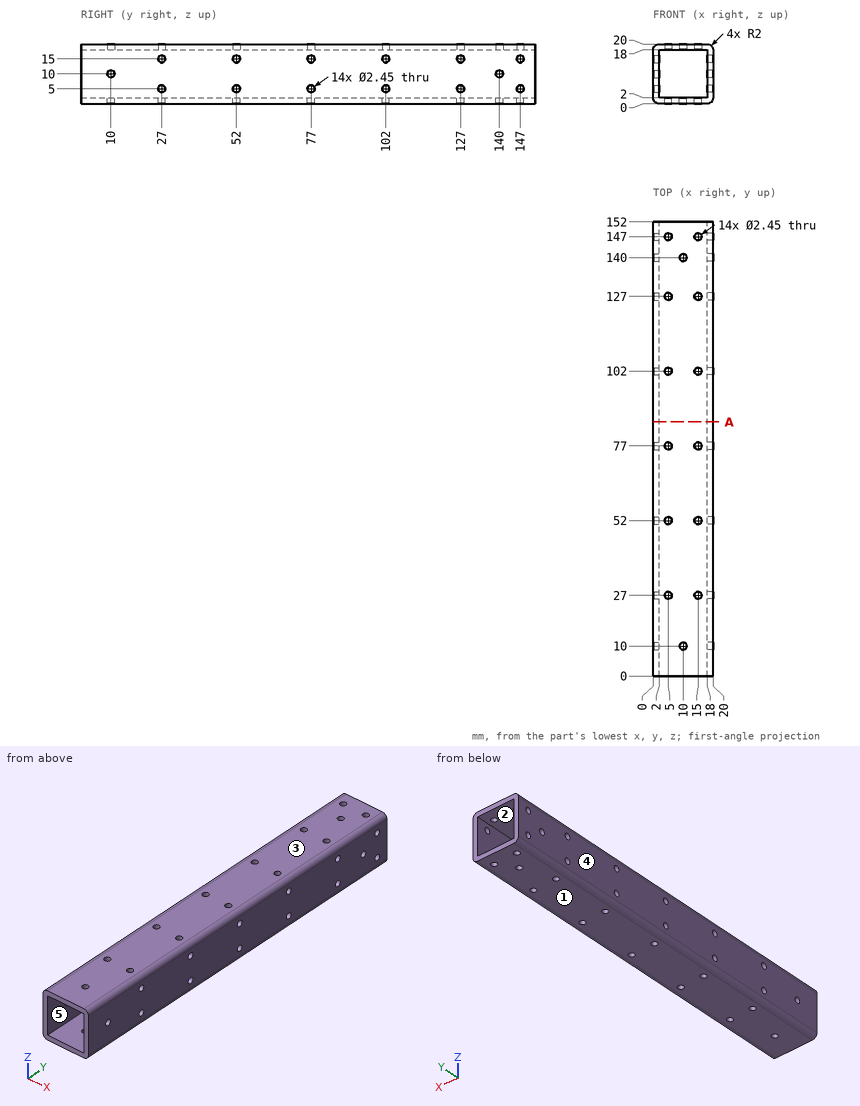
Study the drawing (mm; zero at the part's minimum x, y, z) and answer. A direction names the side the tool comes from. Coordinates: 2 decimals unless noted, no trailing zeros. Write each loop counter-clockwise with the first axis right and the second up, starting at its lowest first coordinate (ties: lowest second). Pieces come first, ordered by that corner, then holes.
Q1. Which of the six approach directions +Z, -Z, +X, -X, +Y, -Y give full straight-line access (tool end or side, diameter ignored) to the marked faces 4 and 5?
Q2. This flat-tipped pin is pushed along its axis until it touches: pin 1 Ø1.5 at (y, z) = (102, 5) entering from +X. Where does it stop, or does it pass through?
Q3. Find the intervals of material crossed by line 1 (Z direction, x = 9, y = 111.5); line 2 (Z direction, x = 0.6, y = 102) (3 decimals), in increasing order.
Q4. Determine the mould class of the marked faces 1, 2 and 3 for opening direction Z: released by +Z, released by -Z, zero draft, split by the parting line, or undercut.
Q5. A cutting plane is placed at A-A, the plane y = 85. Give the vertices of the cut face in (x, z).
Findings below:
1. face 4: +Z, -Z, -X, +Y, -Y
1. face 5: +Y, -Y
2. pin 1: passes through
3. line 1: z = 0 to 2, 18 to 20
3. line 2: z = 0.572 to 3.775, 6.225 to 13.775, 16.225 to 19.428
4. face 1: released by -Z
4. face 2: undercut
4. face 3: released by +Z
5. outline: (0, 2) arc R2 ccw to (2, 0) - (18, 0) arc R2 ccw to (20, 2) - (20, 18) arc R2 ccw to (18, 20) - (2, 20) arc R2 ccw to (0, 18) - close; hole (2, 2) - (18, 2) - (18, 18) - (2, 18) - close
